The listing builds one solid part. Answer for the finished solid, in the listing's coordinates (mm). Give positions to 0.01 mm unless a question says otherwise; leave off trailing zeros. Loops run counter-clockwise (first coordinate to the right, second up) from the corner with the lowest first, then second, coordinate; pieces in that order, holes last. Notation, with made-up numbers: M 30.25,-10.75 L 71.25,-10.75 A19 cw 71.25,-2.75 Z; hole C -36.5,82.25 d9. An arc over 180 degrees is marked long. Return JSON: item names as keys, results as strings.
Autodesk Inventor part; units mm, degrees
ref_plane "YZ Plane" through (0, 0, 0) normal (1, 0, 0) x (0, 1, 0)
ref_plane "XZ Plane" through (0, 0, 0) normal (0, 1, 0) x (-1, 0, 0)
ref_plane "XY Plane" through (0, 0, 0) normal (0, 0, 1) x (1, 0, 0)
sketch "Sketch1" plane through (0, 0, 0) normal (0, 1, 0) x (-1, 0, 0)
  line L0 (0, 0) -> (-127, 0)
  line L1 (-127, 0) -> (-127, 76)
  line L2 (-127, 76) -> (0, 76)
  line L3 (0, 76) -> (0, 0)
  dimension "d0" = 76
  dimension "d1" = 127
extrude "Extrusion1" add sketch "Sketch1" along normal blind 2
sketch "Sketch2" plane through (0, 0, 0) normal (0, -1, 0) x (1, 0, 0)
  line L0 (0, 0) -> (127, 0)
  line L1 (127, 0) -> (127, 76)
  line L2 (127, 76) -> (0, 76)
  line L3 (0, 76) -> (0, 0)
  line L4 (0, 5.4) -> (127, 5.4) construction
  line L5 (0, 38) -> (127, 38) construction
  line L6 (63.5, 76) -> (63.5, 0) construction
  line L7 (121.2, 76) -> (121.2, 0) construction
  line L8 (0, 70.6) -> (127, 70.6) construction
  line L9 (5.8, 76) -> (5.8, 0) construction
  circle A0 centre (121.2, 70.6) radius 2
  circle A1 centre (121.2, 5.4) radius 2
  circle A2 centre (5.8, 70.6) radius 2
  circle A3 centre (5.8, 5.4) radius 2
  dimension "d5" = 32.6
  dimension "d6" = 57.7
  dimension "d7" = 4
extrude "Extrusion2" cut sketch "Sketch2" against normal through all contours A0 | A1 | A2 | A3
sketch "Sketch3" plane through (0, 0, 0) normal (0, -1, 0) x (1, 0, 0)
  line L0 (0, 0) -> (127, 0)
  line L1 (0, 76) -> (0, 0)
  line L2 (10, 93) -> (61, 93)
  line L3 (61, 93) -> (61, 0)
  line L4 (61, 0) -> (10, 0)
  line L5 (10, 0) -> (10, 93)
  line L6 (61, 32) -> (124, 32)
  line L7 (124, 32) -> (124, 67)
  line L8 (124, 67) -> (61, 67)
  line L9 (61, 67) -> (61, 32)
  line L10 (35.5, 93) -> (35.5, 0) construction
  circle A0 centre (35.5, 11) radius 1.5
  circle A1 centre (35.5, 66) radius 1.5
  line L11 (92.5, 67) -> (92.5, 32) construction
  line L12 (124, 49.5) -> (61, 49.5) construction
  circle A2 centre (122, 34.5) radius 1
  circle A3 centre (122, 62.5) radius 1
  circle A4 centre (63.1, 34.5) radius 1
  circle A5 centre (63.1, 62.5) radius 1
  dimension "d10" = 93
  dimension "d12" = 51
  dimension "d13" = 10
  dimension "d14" = 63
  dimension "d15" = 35
  dimension "d16" = 11
  dimension "d17" = 3
  dimension "d20" = 55
  dimension "d25" = 32
  dimension "d26" = 29.5
  dimension "d27" = 2
  dimension "d28" = 15
  dimension "d31" = 28
  dimension "d34" = 58.9
extrude "Extrusion3" cut sketch "Sketch3" against normal through all contours A0 | A1 | A2 | A3 | A4 | A5
properties part number "base_ps"
(1) The part is cut by section B-B (x = 35.5). Determine the outline of the cut face in (y, z).
Values follow:
{"outline": "M 0,0 L 2,0 L 2,9.5 L 0,9.5 Z; M 0,12.5 L 2,12.5 L 2,64.5 L 0,64.5 Z; M 0,67.5 L 2,67.5 L 2,76 L 0,76 Z"}
(2) Determine the mould class of faces 1 (the flat face through (64, 0, 39)), 2 (the cylindrical face through (34.3, 1, 10.1)) for opening direction Z: released by +Z, released by -Z, zero draft, split by the parting line, or undercut.
Values follow:
{"face 1": "zero draft", "face 2": "undercut"}
(3) Straight lines are drawn through the part: line 1 along Z through (x, y) = (35.5, 0.9); line 2 along Z through (x, y) = (121.2, 1.2); line 3 along X through (y, z) = (1.85, 6.5). For each, find the intervals that lie inside material, in ascending order.
Values follow:
{"line 1": "0 to 9.5, 12.5 to 64.5, 67.5 to 76", "line 2": "0 to 3.4, 7.4 to 33.9, 35.1 to 61.9, 63.1 to 68.6, 72.6 to 76", "line 3": "0 to 4.13, 7.47 to 119.53, 122.87 to 127"}
(4) The part is cut by section A-A (z = 5.4). Determine the outline of the cut face in (x, y), and give its area (3 significant figures).
Values follow:
{"outline": "M 0,0 L 3.8,0 L 3.8,2 L 0,2 Z; M 7.8,0 L 119.2,0 L 119.2,2 L 7.8,2 Z; M 123.2,0 L 127,0 L 127,2 L 123.2,2 Z", "area": "238 mm²"}
